For this review, use the dimensioned drawing (mm, ordinates from the lowest corner) and the shaded views. A direction names the side the tool comes from. Round coordinates to 2 decimals unless told otherwise and drop trailing zeros. Loops run counter-clockwise (first coordinate to the right, second up) from the corner with the lowest first, then second, coordinate; pieces in that order, holes last. Notation, with made-up numbers: (-34.5, 60) - (3.5, 60) arc R14 cw to (3.5, 67) - close; hole circle Ø10 at (-37.5, -31). An arc over 180 degrees is marked (long way). Use one line per item in the form item = value. Start each with the question number.
(1) For pin 1 (1.1 mm diameter, centred on x = 11, y = 15.5, fed in from +Z); pin 2 (1.8 mm diameter, centred on y = 15.5, z = 4.5, fed in from +X); pin 3 (2 mm diameter, centred on x = 15.5, z = 3, fed in from +Y), all flat-tipped, find the tip position at first contact; note any pin that passes through.
(2) We need section D-D, the plane x = 9. Write out the cut boundary in (y, z).
(3) Machinability: for the marked faces 5, 6 and 7, which of the approach directions +Z, -Z, +X, -X, +Y, -Y give a long, thin tool a straight path to every point of the face, cutting with its end or side? Answer none if there is none.
(4) Wall thickness on probe 1 along X at (y, z) = (12.25, 3.5); probe 2 along X at (y, z) = (9, 1.7); probe 3 along Z at (x, y) = (10.7, 15): over which ranges is each line inside the solid? List them lowest first. Write a range as [from, to].
(5) The part is to be moulded in two halves that separate along Z. For the marked faces 1, 2, 3 and 4, say which applies: released by +Z, released by -Z, zero draft, split by the parting line, or undercut.
(6) We need section C-C, the plane y = 9. Write out the cut boundary in (x, z), then the cut area to 4 significant figures.
(7) We need section A-A, the plane y = 15. Write out the cut boundary in (x, z).
(8) We need section B-B, the plane z = 3. Write out the cut boundary in (x, y).
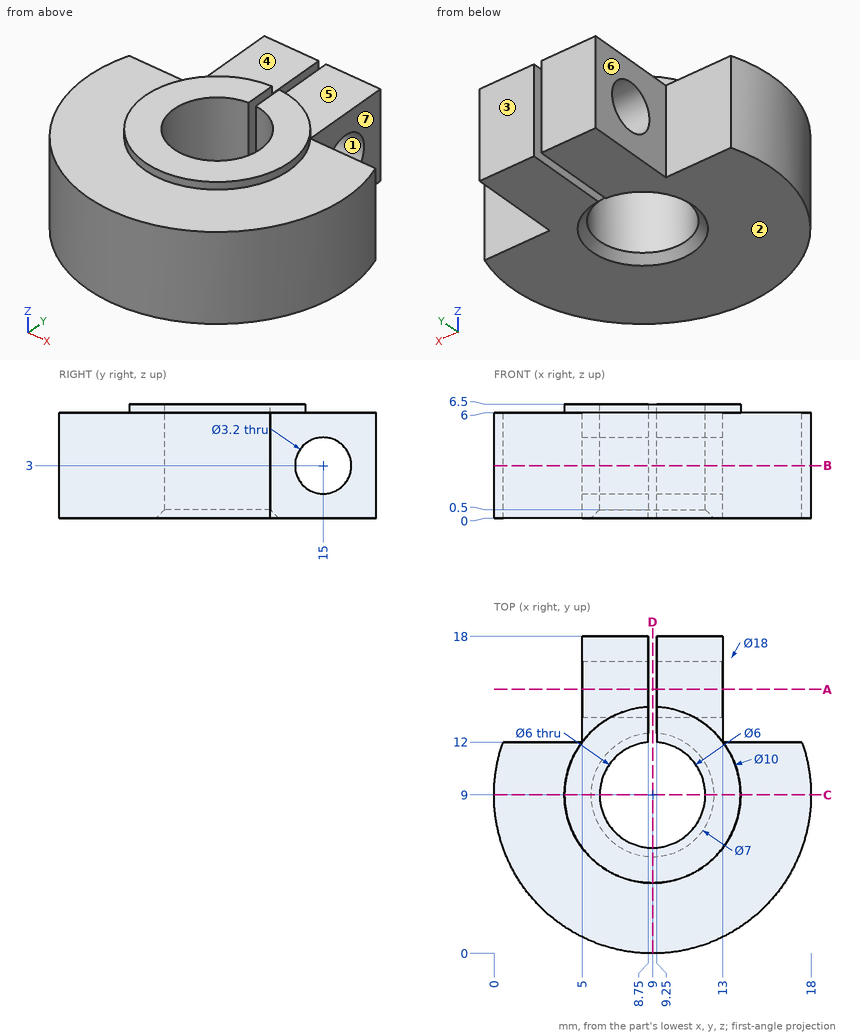
Data:
q1.pin_1 = 6
q1.pin_2 = 13
q1.pin_3 = 12
q2.outline = (0, 0) - (5.5, 0) - (6, 0.5) - (6, 6.5) - (4, 6.5) - (4, 6) - (0, 6) - close
q3.face_5 = +Z, +X, +Y
q3.face_6 = +Z, -Z, -X, +Y
q3.face_7 = +Z, -Z, +X, +Y
q4.probe_1 = [5, 8.75], [9.25, 13]
q4.probe_2 = [0, 6], [12, 18]
q4.probe_3 = [0, 1.4], [4.6, 6]
q5.face_1 = undercut
q5.face_2 = released by -Z
q5.face_3 = zero draft
q5.face_4 = released by +Z
q6.outline = (0, 0) - (5.5, 0) - (6, 0.5) - (6, 6.5) - (4, 6.5) - (4, 6) - (0, 6) - close; (12, 0.5) - (12.5, 0) - (18, 0) - (18, 6) - (14, 6) - (14, 6.5) - (12, 6.5) - close
q6.area = 73.75 mm^2
q7.outline = (5, 0) - (8.75, 0) - (8.75, 1.4) - (5, 1.4) - close; (5, 4.6) - (8.75, 4.6) - (8.75, 6) - (5, 6) - close; (9.25, 0) - (13, 0) - (13, 1.4) - (9.25, 1.4) - close; (9.25, 4.6) - (13, 4.6) - (13, 6) - (9.25, 6) - close
q8.outline = (0.51, 12) arc R9 ccw (long way) to (17.49, 12) - (13, 12) - (13, 13.4) - (9.25, 13.4) - (9.25, 11.99) arc R3 cw (long way) to (8.75, 11.99) - (8.75, 13.4) - (5, 13.4) - (5, 12) - close; (5, 16.6) - (8.75, 16.6) - (8.75, 18) - (5, 18) - close; (9.25, 16.6) - (13, 16.6) - (13, 18) - (9.25, 18) - close
